from build123d import *

# Parameters (mm, degrees)
SKETCH1_W                = 15.3
SKETCH1_H                = 180
SKETCH1_W_2              = 12.3
SKETCH1_H_2              = 20
BOSS_EXTRUDE1_DEPTH      = 120
BOSS_EXTRUDE1_DEPTH_BACK = 9
SKETCH4_R                = 12.5
BOSS_EXTRUDE2_START      = -25
SKETCH6_W                = 40
SKETCH6_H                = 18
SKETCH6_W_2              = 36
SKETCH6_H_2              = 14
BOSS_EXTRUDE2_DEPTH      = 10
SKETCH2_R                = 10.8
CUT_EXTRUDE1_DEPTH       = 199
SKETCH5_R                = 11
CUT_EXTRUDE2_DEPTH       = 133
SKETCH7_W                = 36
SKETCH7_H                = 14
CUT_EXTRUDE3_DEPTH       = 15
BOSS_EXTRUDE3_START      = -11
SKETCH8_W                = 5.5
SKETCH8_H                = 22
BOSS_EXTRUDE3_DEPTH      = 6
SKETCH10_W               = 23.5
SKETCH10_H               = 16.6
SKETCH10_W_2             = 19.5
SKETCH10_H_2             = 12.6
BOSS_EXTRUDE5_DEPTH      = 10
SKETCH11_W               = 19.5
SKETCH11_H               = 12.6
CUT_EXTRUDE4_DEPTH       = 12
SKETCH13_W               = 40
SKETCH13_H               = 18
SKETCH13_R               = 5
BOSS_EXTRUDE6_DEPTH      = 1
CUT_EXTRUDE7_DEPTH       = 106
CUT_EXTRUDE7_DEPTH_BACK  = 39
SKETCH15_W               = 30.6
SKETCH15_H               = 203.669908639
SKETCH16_R               = 12.5
BOSS_EXTRUDE7_DEPTH      = 2
SKETCH17_R               = 11.5
SKETCH17_R_2             = 10
BOSS_EXTRUDE8_DEPTH      = 20
CUT_EXTRUDE8_START       = -2
SKETCH18_R               = 10
CUT_EXTRUDE8_DEPTH       = 2
SKETCH9_R                = 1.75
BOSS_EXTRUDE4_DEPTH      = 2
CUT_EXTRUDE10_DEPTH      = 182


with BuildPart() as part:
    # Sketch1 → Revolve1 (revolve)
    with BuildSketch(Plane.XY, mode=Mode.PRIVATE) as revolve1_sk:
        with Locations((-7.65, 90)):
            Rectangle(SKETCH1_W, SKETCH1_H)
        with Locations((-6.15, -10)):
            Rectangle(SKETCH1_W_2, SKETCH1_H_2)
    revolve(revolve1_sk.sketch.rotate(Axis((0, 259.808396335, 0), (0, -1, 0)), 270), axis=Axis((0, 259.808396335, 0), (0, -1, 0)))

    # Sketch4 → Boss-Extrude1 (add, two sides: drawn at the far end of the back side and taken through both)
    with BuildSketch(Plane.XY.offset(15.3).offset(-BOSS_EXTRUDE1_DEPTH_BACK)):
        with Locations((0, 152.071263422)):
            Circle(SKETCH4_R)
    extrude(amount=BOSS_EXTRUDE1_DEPTH + BOSS_EXTRUDE1_DEPTH_BACK)

    # Sketch6 → Boss-Extrude2 (add)
    with BuildSketch(Plane.ZY.offset(12.5).offset(BOSS_EXTRUDE2_START)):
        with Locations((89.3, 152.071263422)):
            Rectangle(SKETCH6_W, SKETCH6_H)
        with Locations((89.3, 152.071263422)):
            Rectangle(SKETCH6_W_2, SKETCH6_H_2, mode=Mode.SUBTRACT)
    extrude(amount=BOSS_EXTRUDE2_DEPTH)

    # Sketch2 → Cut-Extrude1 (cut)
    with BuildSketch(Plane.XZ.offset(20)):
        with Locations(Location((0, 0, 0), (0, 0, 270))):
            Circle(SKETCH2_R)
    extrude(amount=-CUT_EXTRUDE1_DEPTH, mode=Mode.SUBTRACT)

    # Sketch5 → Cut-Extrude2 (cut)
    with BuildSketch(Plane.XY.offset(135.3)):
        with Locations((0, 152.071263422)):
            Circle(SKETCH5_R)
    extrude(amount=-CUT_EXTRUDE2_DEPTH, mode=Mode.SUBTRACT)

    # Sketch7 → Cut-Extrude3 (cut)
    with BuildSketch(Plane(origin=(12.5, 0, 0), x_dir=(0, 0, -1), z_dir=(1, 0, 0))):
        with Locations((-89.3, 152.071263422)):
            Rectangle(SKETCH7_W, SKETCH7_H)
    extrude(amount=-CUT_EXTRUDE3_DEPTH, mode=Mode.SUBTRACT)

    # Sketch8 → Boss-Extrude3 (add)
    with BuildSketch(Plane.XY.offset(71.3).offset(BOSS_EXTRUDE3_START)):
        with Locations((2.75, 152.071263422)):
            Rectangle(SKETCH8_W, SKETCH8_H)
        with BuildLine():
            ThreePointArc((8.485281374, 159.071263422), (7.105810702, 160.468135117), (5.5, 161.597542863))
            Line((5.5, 161.597542863), (5.5, 142.54498398))
            ThreePointArc((5.5, 142.54498398), (7.105810702, 143.674391726), (8.485281374, 145.071263422))
            ThreePointArc((8.485281374, 145.071263422), (11, 152.071263422), (8.485281374, 159.071263422))
        make_face()
    extrude(amount=-BOSS_EXTRUDE3_DEPTH)

    # Sketch10 → Boss-Extrude5 (add)
    with BuildSketch(Plane(origin=(12.5, 0, 0), x_dir=(0, 0, -1), z_dir=(1, 0, 0))):
        with Locations((-121.55, 152.071263422)):
            Rectangle(SKETCH10_W, SKETCH10_H)
        with Locations((-121.55, 152.071263422)):
            Rectangle(SKETCH10_W_2, SKETCH10_H_2, mode=Mode.SUBTRACT)
    extrude(amount=-BOSS_EXTRUDE5_DEPTH)

    # Sketch11 → Cut-Extrude4 (cut)
    with BuildSketch(Plane(origin=(12.5, 0, 0), x_dir=(0, 0, -1), z_dir=(1, 0, 0))):
        with Locations((-121.55, 152.071263422)):
            Rectangle(SKETCH11_W, SKETCH11_H)
    extrude(amount=-CUT_EXTRUDE4_DEPTH, mode=Mode.SUBTRACT)

    # Sketch13 → Boss-Extrude6 (add)
    with BuildSketch(Plane(origin=(12.5, 0, 0), x_dir=(0, 0, -1), z_dir=(1, 0, 0))):
        with Locations((-89.3, 152.071263422)):
            Rectangle(SKETCH13_W, SKETCH13_H)
        with Locations((-100.8, 152.071263422)):
            Circle(SKETCH13_R, mode=Mode.SUBTRACT)
        with Locations((-77.8, 152.071263422)):
            Circle(SKETCH13_R, mode=Mode.SUBTRACT)
    extrude(amount=BOSS_EXTRUDE6_DEPTH)

    # Sketch15 → Cut-Extrude7 (cut, two sides: drawn at the far end of the back side and taken through both)
    with BuildSketch(Plane(origin=(0, 0, 0), x_dir=(0, 0, -1), z_dir=(1, 0, 0)).offset(-CUT_EXTRUDE7_DEPTH_BACK)):
        with Locations((0, 78.165045681)):
            Rectangle(SKETCH15_W, SKETCH15_H)
    extrude(amount=CUT_EXTRUDE7_DEPTH + CUT_EXTRUDE7_DEPTH_BACK, mode=Mode.SUBTRACT)

    # Sketch16 → Boss-Extrude7 (add)
    with BuildSketch(Plane(origin=(0, 0, 15.3), x_dir=(-1, 0, 0), z_dir=(0, 0, -1))):
        with Locations(Location((0, 152.071263422, 0), (0, 0, 180))):
            Circle(SKETCH16_R)
    extrude(amount=-BOSS_EXTRUDE7_DEPTH)

    # Sketch17 → Boss-Extrude8 (add)
    with BuildSketch(Plane(origin=(0, 0, 15.3), x_dir=(-1, 0, 0), z_dir=(0, 0, -1))):
        with Locations((0, 152.071263422)):
            Circle(SKETCH17_R)
        with Locations((0, 152.071263422)):
            Circle(SKETCH17_R_2, mode=Mode.SUBTRACT)
    extrude(amount=BOSS_EXTRUDE8_DEPTH)

    # Sketch18 → Cut-Extrude8 (cut)
    with BuildSketch(Plane(origin=(0, 0, 15.3), x_dir=(-1, 0, 0), z_dir=(0, 0, -1)).offset(CUT_EXTRUDE8_START)):
        with Locations((0, 152.071263422)):
            Circle(SKETCH18_R)
    extrude(amount=CUT_EXTRUDE8_DEPTH, mode=Mode.SUBTRACT)

    # Sketch9 → Boss-Extrude4 (add)
    with BuildSketch(Plane.ZY):
        with Locations((57.05, 159.671263422)):
            Circle(SKETCH9_R)
        with Locations(Location((57.05, 144.471263422, 0), (0, 0, 180))):
            Circle(SKETCH9_R)
    extrude(amount=BOSS_EXTRUDE4_DEPTH)

    # Sketch19 → Cut-Extrude10 (cut)
    with BuildSketch(Plane.XY.offset(135.3)):
        with BuildLine():
            ThreePointArc((0, 141.071263422), (-11, 152.071263422), (0, 163.071263422))
            Line((0, 163.071263422), (0, 164.571263422))
            ThreePointArc((0, 164.571263422), (-12.5, 152.071263422), (0, 139.571263422))
            Line((0, 139.571263422), (0, 141.071263422))
        make_face()
        with BuildLine():
            Line((-2.177257281, 161.7010227), (0, 161.7010227))
            Line((0, 161.7010227), (0, 163.071263422))
            ThreePointArc((0, 163.071263422), (-11, 152.071263422), (0, 141.071263422))
            Line((0, 141.071263422), (0, 142.542341384))
            Line((0, 142.542341384), (-2.177257281, 142.542341384))
            Line((-2.177257281, 142.542341384), (-2.177257281, 143.338591967))
            ThreePointArc((-2.177257281, 143.338591967), (-9, 152.071263422), (-2.177257281, 160.803934876))
            Line((-2.177257281, 160.803934876), (-2.177257281, 161.7010227))
        make_face()
        with BuildLine():
            Line((-2.177257281, 143.338591967), (-2.177257281, 160.803934876))
            ThreePointArc((-2.177257281, 160.803934876), (-9, 152.071263422), (-2.177257281, 143.338591967))
        make_face()
    extrude(amount=-CUT_EXTRUDE10_DEPTH, mode=Mode.SUBTRACT)


solid = part.part
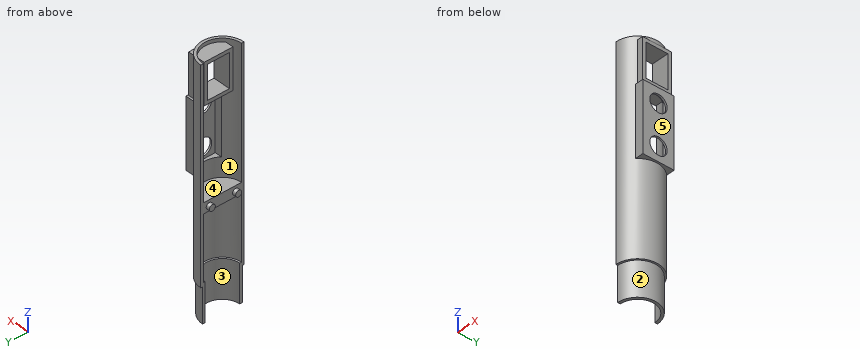
The model under review builds one solid part; all positions refer to its coordinate system, in mm. Face numbers are marked on the shaded views. A direction names the side the tool comes from. Round coordinates to 2 decimals unless told otherwise and drop trailing zeros. Loops run counter-clockwise (first coordinate to the right, second up) from the corner with the lowest first, then second, coordinate; pieces in that order, holes last. Notation, with made-up numbers: (-21.75, -35.5) -> (6.25, -35.5) arc R12 ccw to (6.25, -30.5) -> close; hole circle Ø4 at (19, 71). An arc over 180 degrees is marked (long way). Write item = value, one per line. Start each with the question number.
Item 1: Take a section at C-C on z = 100.8. Give the boundary of the cut face in (x, y), plus the area to 3 significant figures.
Item 2: Take a section at B-B on z = 57.05. Give the boundary of the cut face in (x, y).
Item 3: Take a section at D-D on y = 149. Count the separate pieces of the cut face and the enclosed holes in it, plus the area to 3 significant figures.
Item 4: Insertion check: pin 1 (1.5 mm diameter, centred on y = 143.5, z = 109.5, fed in from +X); pin 2 (8 mm diameter, centred on x = 6, z = 125, fed in from +Y); pin 3 (3 mm diameter, centred on x = 10, z = 98, fed in from -Y); pin 4 (1.4 mm diameter, centred on x = 12, z = 81.5, fed in from +Y). Each pin has a flat end and moves straight along its axis. Give the tip position at first contact, or say it passes through.
Item 5: To check wall thickness, follow L1, parallel to Z at x = 5, y = 148; L2, parallel to Y at x = 13, z = 77.8; L3, parallel to Z at x = 2, y = 148.25. State the ranges of each line that lie inside material, in increasing order.
Item 6: Take a section at A-A on z = 119.5. Give the boundary of the cut face in (x, y).
Item 7: Mouldability with a two-part tool opening along Z and no side actions: class the marked faces 1 and 2 as released by +Z, released by -Z, zero draft, split by the parting line, or undercut.
Item 8: For the marked faces 3, 4 and 5, list the 3-axis set-ups (+Z, -Z, +X, -X, +Y, -Y) from which the entire face can be reached by the end or side of a thin tool; tool diameter is ignored.
Result:
q1.outline = (0, 139.57) arc R12.5 ccw to (8.67, 143.07) -> (13.5, 143.07) -> (13.5, 147.07) -> (12.5, 147.07) -> (12.5, 145.07) -> (8.49, 145.07) arc R11 cw to (0, 141.07) -> close; (0, 163.07) arc R11 cw to (8.49, 159.07) -> (12.5, 159.07) -> (12.5, 157.07) -> (13.5, 157.07) -> (13.5, 161.07) -> (8.67, 161.07) arc R12.5 ccw to (0, 164.57) -> close
q1.area = 52.6 mm²
q2.outline = (-2, 142.72) -> (0, 142.72) -> (0, 139.57) arc R12.5 ccw to (0, 164.57) -> (0, 161.42) -> (-2, 161.42) -> (-2, 157.92) -> (0, 157.92) -> (0, 146.22) -> (-2, 146.22) -> close
q3.separate_pieces = 4
q3.enclosed_holes = 0
q3.area = 257 mm²
q4.pin_1 = 13.5
q4.pin_2 = 164.41
q4.pin_3 = 142.91
q4.pin_4 = 161.07
q5.L1 = 54.3 to 60.3, 109.8 to 111.8, 131.3 to 133.3
q5.L2 = 143.07 to 147.07, 157.07 to 161.07
q5.L3 = 54.3 to 60.3
q6.outline = (0, 139.57) arc R12.5 ccw to (9.35, 143.77) -> (12.5, 143.77) -> (12.5, 145.77) -> (2.5, 145.77) -> (2.5, 143.77) -> (7.22, 143.77) arc R11 cw to (0, 141.07) -> close; (0, 163.07) arc R11 cw to (7.22, 160.37) -> (2.5, 160.37) -> (2.5, 158.37) -> (12.5, 158.37) -> (12.5, 160.37) -> (9.35, 160.37) arc R12.5 ccw to (0, 164.57) -> close
q7.face_1 = undercut
q7.face_2 = zero draft
q8.face_3 = -Z, -X
q8.face_4 = -X
q8.face_5 = +Z, -Z, +X, +Y, -Y
